```python
from build123d import *

# Parameters (mm, degrees)
SKETCH1_W           = 52
SKETCH1_H           = 40
BOSS_EXTRUDE1_DEPTH = 3
SKETCH2_W           = 35
SKETCH2_H           = 7
BOSS_EXTRUDE2_DEPTH = 40
CUT_EXTRUDE1_DEPTH  = 56.472966389
SKETCH4_W           = 52
SKETCH4_H           = 40
BOSS_EXTRUDE3_DEPTH = 31
CUT_EXTRUDE10_DEPTH = 93.628289415
CUT_EXTRUDE11_DEPTH = 93.628289415
SKETCH8_R           = 5
BOSS_EXTRUDE4_DEPTH = 3
SKETCH9_R           = 1
BOSS_EXTRUDE5_DEPTH = 31
SKETCH10_W          = 43.211860489
SKETCH10_H          = 44.174227803
CUT_EXTRUDE12_DEPTH = 70


with BuildPart() as part:
    # Sketch1 → Boss-Extrude1 (new body)
    with BuildSketch(Plane(origin=(0, 0, 0), x_dir=(1, 0, 0), z_dir=(0, 1, 0))):
        Rectangle(SKETCH1_W, SKETCH1_H)
    extrude(amount=BOSS_EXTRUDE1_DEPTH)

    # Sketch2 → Boss-Extrude2 (add)
    with BuildSketch(Plane(origin=(0, 3, 0), x_dir=(1, 0, 0), z_dir=(0, 1, 0))):
        with Locations((1.5, 0)):
            Rectangle(SKETCH2_W, SKETCH2_H)
    extrude(amount=BOSS_EXTRUDE2_DEPTH)

    # Sketch3 → Cut-Extrude1 (cut, through all)
    with BuildSketch(Plane(origin=(0, 0, -3.5), x_dir=(-1, 0, 0), z_dir=(0, 0, -1))):
        Polygon((1, 43), (16, 3), (16, 43), align=None)
    extrude(amount=-CUT_EXTRUDE1_DEPTH, mode=Mode.SUBTRACT)

    # Sketch4 → Boss-Extrude3 (add)
    with BuildSketch(Plane(origin=(0, 43, 0), x_dir=(1, 0, 0), z_dir=(0, 1, 0))):
        Rectangle(SKETCH4_W, SKETCH4_H)
    extrude(amount=BOSS_EXTRUDE3_DEPTH)

    # Sketch5 → Cut-Extrude10 (cut, through all)
    with BuildSketch(Plane.ZY.offset(26)):
        with BuildLine():
            Line((-20, 43), (-20, 74))
            Line((-20, 74), (0, 74))
            ThreePointArc((0, 74), (-15.399591999, 60.261410302), (-3.5, 43.400331129))
            Line((-3.5, 43.400331129), (-3.5, 43))
            Line((-3.5, 43), (-20, 43))
        make_face()
    extrude(amount=-CUT_EXTRUDE10_DEPTH, mode=Mode.SUBTRACT)

    # Sketch7 → Cut-Extrude11 (cut, through all)
    with BuildSketch(Plane.ZY.offset(26)):
        with BuildLine():
            Line((0, 74), (20, 74))
            Line((20, 74), (20, 43))
            Line((20, 43), (3.5, 43))
            Line((3.5, 43), (3.5, 43.400331129))
            ThreePointArc((3.5, 43.400331129), (15.399591999, 60.261410302), (0, 74))
        make_face()
    extrude(amount=-CUT_EXTRUDE11_DEPTH, mode=Mode.SUBTRACT)

    # Sketch8 → Boss-Extrude4 (add)
    with BuildSketch(Plane.ZY.offset(26)):
        with Locations(Location((0, 58.5, 0), (0, 0, 180))):
            Circle(SKETCH8_R)
    extrude(amount=BOSS_EXTRUDE4_DEPTH)

    # Sketch9 → Boss-Extrude5 (add)
    with BuildSketch(Plane.ZY.offset(29)):
        with Locations((0, 58.5)):
            Circle(SKETCH9_R)
    extrude(amount=BOSS_EXTRUDE5_DEPTH)

    # Sketch10 → Cut-Extrude12 (cut)
    with BuildSketch(Plane.ZY.offset(-30)):
        with Locations((-0.422313508, 21.268278388)):
            Rectangle(SKETCH10_W, SKETCH10_H)
    extrude(amount=CUT_EXTRUDE12_DEPTH, mode=Mode.SUBTRACT)


solid = part.part
```
Model file for the job. Use its own axes, mm. A direction names the side the tool comes from. Round coordinates to 2 decimals unless told otherwise and drop trailing zeros. Write each loop counter-clockwise with the first axis right and the second up, starting at its lowest first coordinate (ties: lowest second). Pieces come first, ordered by that corner, then holes. Notation, with made-up numbers: M 23,-23 L 61,-23 A10 cw 61,-6 Z; hole C -7.5,15.5 d3. An arc over 180 degrees is marked long. Put each result on its own line as item: value.
Item 1: Probe L1, parallel to X at y = 48.5, z = 9.5; L2, parallel to X at y = 62.5, z = 0.5; L3, parallel to Y at x = -17.5, z = -1.5. List the from-to ranges inside material, lowest first. Write a range as from..to.
Responses:
L1: -26..26
L2: -29..26
L3: 43.36..73.93
Item 2: Cut at A-A (y = 58.5). List the corners of the cut face in (x, z), and give its area (3 significant figures).
Responses:
outline: M -60,-1 L -29,-1 L -29,-5 L -26,-5 L -26,-15.5 L 26,-15.5 L 26,15.5 L -26,15.5 L -26,5 L -29,5 L -29,1 L -60,1 Z
area: 1,700 mm²
Item 3: Cut at B-B (x = 15.5). List the corners of the cut face in (y, z).
Responses:
outline: M 43.36,-3.5 L 43.4,-3.5 A15.5 ccw long 43.4,3.5 L 43.36,3.5 Z
Item 4: Cut at D-D (x = -47). List the corners of the cut face in (y, z).
Responses:
outline: C 58.5,0 d2
Item 5: Cut at C-C (z = 6). List the corners of the cut face in (x, y), and give its area (3 significant figures).
Responses:
outline: M -26,44.21 L 26,44.21 L 26,72.79 L -26,72.79 Z
area: 1,490 mm²
Item 6: Tool access for faces 1 (the cylindrical face through (-44.28, 59.34, 0.54)), 2 (the flat face through (0, 43.355, 0)): list every direction of +Z, -Z, +X, -X, +Y, -Y with a clear straight run to the whole face (end or side of a thin tool).
Responses:
face 1: -X
face 2: +Z, -Z, +X, -X, -Y
Item 7: Flat gauge pins, fed straight in: P1, Ø10, axis at y = 63, z = -11.5, coming from the -X side; P2, Ø3, axis at x = 6.5, z = 10, coming from the +Y side; P3, Ø2, axis at x = -7, z = -10, coming from the -Y side. Where does each tip first touch, or does it go through?
Responses:
P1: x = -26
P2: y = 71.46
P3: y = 45.88
